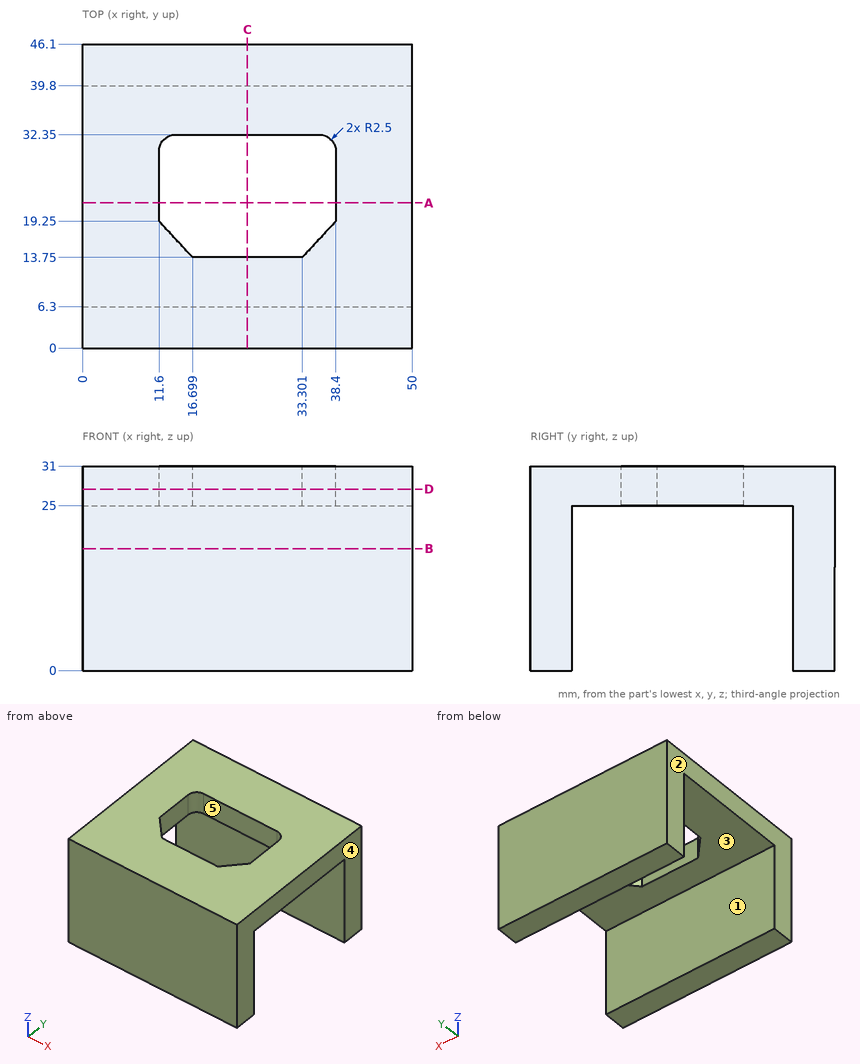
Job drawing, mm, ordinate dimensions from the low corner. One solid piece. A direction names the side the tool comes from. Coordinates: 2 decimals unless noted, no trailing zeros. Write each loop counter-clockwise with the first axis right and the second up, starting at its lowest first coordinate (ties: lowest second). Pieces come first, ordered by that corner, then holes. Notation, with made-up numbers: M 79.25,82.5 L 100.25,82.5 A8 ccw 100.25,92.5 Z; hole C 16,-8 d5. An arc over 180 degrees is marked long. Answer as a JSON object with one key per item and string values. Group by question number.
1) Saw through at D-D (z = 27.5). Write the cut outline in (x, y), plus the area to 3 significant figures.
2) Pin check, flat tip, straight feed: pin 1 Ø8 at (x, y) = (40.5, 18) entering from -Z. Stop position of the tip, or through.
3) Saw through at C-C (x = 25). Write the cut outline in (y, z), plus the area to 3 significant figures.
4) Wall check: line 1 (Y direction, x = 20.5, z = 6.5); line 2 (Y direction, x = 24.5, z = 28); line 3 (X direction, y = 26, z = 28). Give the ranges that are in metal, low to high. Write a range as from..to.
5) Mould opens along X. For the marked faces 3, 4 and 5 say: +X half, -X half, draft (parallel to the pull), parting line (faces both ways), or undercut.
6) Saw through at A-A (y = 22). Write the cut outline in (x, z), plus the area to 3 significant figures.
7) Tool access for the marked faces 1 and 2: list every direction of +Z, -Z, +X, -X, +Y, -Y with a clear straight run to the whole face (end or side of a thin tool).
8) Saw through at B-B (z = 18.5). Write the cut outline in (x, y), plus the area to 3 significant figures.
Values follow:
{
 "1": {"outline": "M 0,0 L 50,0 L 50,46.1 L 0,46.1 Z; hole M 11.6,19.25 L 16.7,13.75 L 33.3,13.75 L 38.4,19.25 L 38.4,29.85 A2.5 ccw 35.9,32.35 L 14.1,32.35 A2.5 ccw 11.6,29.85 Z", "area": "1,840 mm2"},
 "2": {"pin 1": "stops at z = 25"},
 "3": {"outline": "M 0,0 L 6.3,0 L 6.3,25 L 13.75,25 L 13.75,31 L 0,31 Z; M 32.35,25 L 39.8,25 L 39.8,0 L 46.1,0 L 46.1,31 L 32.35,31 Z", "area": "480 mm2"},
 "4": {"line 1": "y = 0..6.3, 39.8..46.1", "line 2": "y = 0..13.75, 32.35..46.1", "line 3": "x = 0..11.6, 38.4..50"},
 "5": {"face 3": "draft", "face 4": "+X half", "face 5": "undercut"},
 "6": {"outline": "M 0,25 L 11.6,25 L 11.6,31 L 0,31 Z; M 38.4,25 L 50,25 L 50,31 L 38.4,31 Z", "area": "139 mm2"},
 "7": {"face 1": "-Z, +X, -X", "face 2": "+Z, -Z, -X, +Y, -Y"},
 "8": {"outline": "M 0,0 L 50,0 L 50,6.3 L 0,6.3 Z; M 0,39.8 L 50,39.8 L 50,46.1 L 0,46.1 Z", "area": "630 mm2"}
}
